Can you work these out from the model? Positions are in its coordinate system, mm. Round coordinates to 2 decimals unless told otherwise and drop trailing zeros. Write each loop counter-clockwise with the first axis right and the second up, starting at its lowest first coordinate (ties: lowest second). Pieces come first, ordered by that corner, then holes. Notation, with made-up numbers: M 23,66 L 55,66 A3 cw 55,71 Z; hole C 28.25,83 d7. An arc over 180 degrees is marked long. Answer in a Markdown table with one row per item. Add a question column.
(1) Suppose I cut it at A-A, the plane x = 12.75. Write out the boundary of the cut face in (y, z).
(2) I'm going to push flat-ended pins straight in: pin 1 (0.9 mm diameter, centred on y = 0.5, z = -31, fed in from +X); pin 2 (1.9 mm diameter, centred on x = 12, y = -0.5, fed in from +Z). Where does each tip first touch, or does it pass through?
(3) If I drill on probe 1 along X at (y, z) = (-0.1, -44); probe 2 along Z at (x, y) = (16.25, -0.35); probe 3 along X at (y, z) = (1, -42), over which ranges is the centre line in solid material (lowest first)?
(4) Suppose I cut it at C-C, the plane y = -0.3. Write out the boundary of the cut face in (x, z).
(5) Suppose I cut it at B-B, the plane z = -46.5. Write out the boundary of the cut face in (x, y).
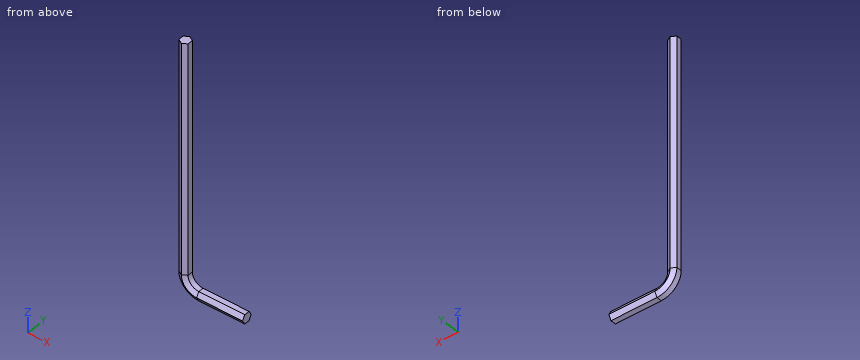
from build123d import *


with BuildPart() as part:
    # Sweep1: sweep along a path in Sketch2
    with BuildLine(Plane(origin=(0, 0, 0), x_dir=(1, 0, 0), z_dir=(0, 1, 0))) as sweep1_path:
        Line((0, 0), (0, 75))
        ThreePointArc((0, 75), (1.464466094, 78.535533906), (5, 80))
        Line((5, 80), (20, 80))
    # Sketch1 → Sweep1 (sweep)
    with BuildSketch(Plane.XY):
        Polygon((-1.5, 0.866025404), (-1.5, -0.866025404), (0, -1.732050808), (1.5, -0.866025404), (1.5, 0.866025404), (0, 1.732050808), align=None)
    sweep(path=sweep1_path.line)


solid = part.part
Calculated:
| question | item | result |
|---|---|---|
| 1 | outline | M -1.73,-80 L -0.87,-81.5 L 0.87,-81.5 L 1.73,-80 L 0.87,-78.5 L -0.87,-78.5 Z |
| 2 | pin 1 | x = 1.5 |
| 2 | pin 2 | z = -78.5 |
| 3 | probe 1 | -1.5 to 1.5 |
| 3 | probe 2 | -81.5 to -78.5 |
| 3 | probe 3 | -1.27 to 1.27 |
| 4 | outline | M -1.5,-75 A6.5 ccw 5,-81.5 L 20,-81.5 L 20,-78.5 L 5,-78.5 A3.5 cw 1.5,-75 L 1.5,0 L -1.5,0 Z |
| 5 | outline | M -1.5,-0.87 L 0,-1.73 L 1.5,-0.87 L 1.5,0.87 L 0,1.73 L -1.5,0.87 Z |
